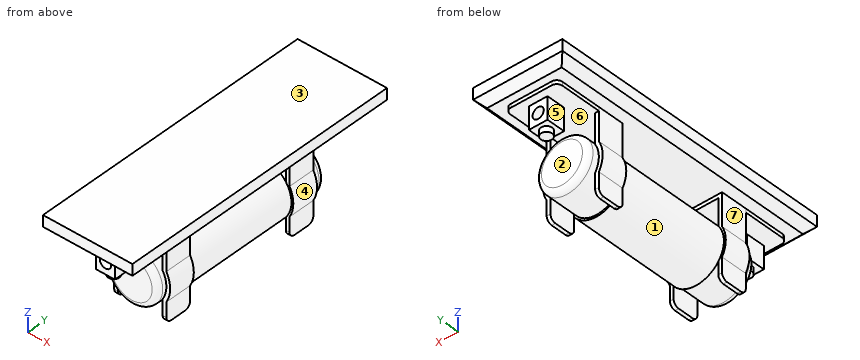
Solid Edge part; units mm, degrees
sketch "Sketch1" plane through (0, 0, 0) normal (0, -1, 0) x (1, 0, 0)
  circle A0 centre (-33.5391, 14.6196) radius 7.5
extrude "Protrusion1" add sketch "Sketch1" against normal blind 30
sketch "Sketch2" plane through (-33.5391, 0, 14.6196) normal (0, -1, 0) x (1, 0, 0)
  circle A0 centre (0, 0) radius 7
extrude "ExtrudedProtrusion_2" add sketch "Sketch2" along normal blind 9.75 and the other way blind 40.4
fillet "Round_1" radius 1.5 2 edges at (-40.5391, -9.75, 14.6196) (-40.5391, 40.4, 14.6196)
sketch "Sketch3" plane through (-33.5391, 30, 14.6196) normal (0, 1, 0) x (1, 0, 0)
  line L0 (-6, -11.6345) -> (-6, -3.6056)
  arc A0 (-6, -3.6056) -> (-6, 3.6056) centre (0, 0) cw
  line L1 (-6, 3.6056) -> (-6, 9.3463)
  line L2 (-7, 9.3463) -> (-6, 9.3463)
  line L3 (-7, 3.873) -> (-7, 9.3463)
  arc A1 (-7, -3.873) -> (-7, 3.873) centre (0, 0) cw
  line L4 (-7, -12.6345) -> (-7, -3.873)
  line L5 (7, -12.6345) -> (-7, -12.6345)
  line L6 (7, -3.873) -> (7, -12.6345)
  arc A2 (7, 3.873) -> (7, -3.873) centre (0, 0) cw
  line L7 (7, 9.3463) -> (7, 3.873)
  line L8 (6, 9.3463) -> (7, 9.3463)
  line L9 (6, 3.6056) -> (6, 9.3463)
  line L10 (6, -11.6345) -> (6, -3.6056)
  line L11 (-6, -11.6345) -> (6, -11.6345)
  arc A3 (6, 3.6056) -> (6, -3.6056) centre (0, 0) cw
extrude "ExtrudedProtrusion_3" add sketch "Sketch3" along normal blind 7.1438
sketch "Sketch4" plane through (-33.5391, 37.1438, 16.2637) normal (0, 1, 0) x (1, 0, 0)
  line L0 (7, -9.9904) -> (-7, -9.9904)
  line L1 (-7, -9.9904) -> (-7, -10.9904)
  line L2 (-7, -10.9904) -> (7, -10.9904)
  line L3 (7, -10.9904) -> (7, -9.9904)
extrude "ExtrudedProtrusion_4" add sketch "Sketch4" along normal blind 12.5
fillet "Round_2" radius 1.5 6 edges at (-40.0391, 37.1438, 5.2733) (-40.0391, 30, 5.2733) (-27.0391, 30, 5.2733) (-27.0391, 37.1438, 5.2733) (-26.5391, 49.6437, 26.7541) (-40.5391, 49.6437, 26.7541)
mirror "Mirror1" about plane through (0, 15, 0) normal (0, -1, 0) of "ExtrudedProtrusion_4", "ExtrudedProtrusion_3"
fillet "Round1" radius 1.5 6 edges at (-40.0391, -7.1438, 5.2733) (-40.0391, 0, 5.2733) (-27.0391, 0, 5.2733) (-27.0391, -7.1438, 5.2733) (-26.5391, -19.6438, 26.7541) (-40.5391, -19.6438, 26.7541)
sketch "Sketch5" plane through (-33.5391, 49.8219, 27.2541) normal (0, 0, 1) x (1, 0, 0)
  line L0 (12, 3.928) -> (12, -72.823)
  line L1 (12, -72.823) -> (-12, -72.823)
  line L2 (-12, 3.928) -> (-12, -72.823)
  line L3 (-12, 3.928) -> (12, 3.928)
  dimension "D1" = 12
extrude "ExtrudedProtrusion_7" add sketch "Sketch5" along normal blind 5
chamfer "Chamfer_1" distance 2 angle 45 4 edges at (-33.5391, 53.7499, 27.2541) (-45.5391, 15.3744, 27.2541) (-33.5391, -23.0011, 27.2541) (-21.5391, 15.3744, 27.2541)
sketch "Sketch6" plane through (-33.5391, 39.8219, 26.2541) normal (0, 0, -1) x (0, -1, 0)
  line L0 (-7.7578, -2.5) -> (-2.7578, -2.5)
  line L1 (-2.7578, -2.5) -> (-2.7578, 2.5)
  line L2 (-2.7578, 2.5) -> (-7.7578, 2.5)
  line L3 (-7.7578, 2.5) -> (-7.7578, -2.5)
  line L4 (52.4656, -2.5) -> (57.4656, -2.5)
  line L5 (57.4656, -2.5) -> (57.4656, 2.5)
  line L6 (57.4656, 2.5) -> (52.4656, 2.5)
  line L7 (52.4656, 2.5) -> (52.4656, -2.5)
extrude "ExtrudedProtrusion_8" add sketch "Sketch6" along normal blind 6
sketch "Sketch7" plane through (-33.5391, 47.5797, 22.7541) normal (0, 1, 0) x (1, 0, 0)
  circle A0 centre (0, -0.5) radius 1.5
extrude "Cutout1" cut sketch "Sketch7" against normal up to next
sketch "Sketch8" plane through (-33.5391, -17.6438, 22.7541) normal (0, -1, 0) x (-1, 0, 0)
  circle A0 centre (0, -0.5) radius 1.5
extrude "Cutout2" cut sketch "Sketch8" against normal up to next
sketch "Sketch9" plane through (-33.5391, 45.0797, 20.2541) normal (0, 0, -1) x (0, 1, 0)
  circle A0 centre (0, 0) radius 1.5
  circle A1 centre (-60.2235, 0) radius 1.5
extrude "ExtrudedProtrusion_9" add sketch "Sketch9" along normal blind 1.5
Part model, mm, in its own coordinate system. Face numbers are marked on the shaded views. A direction names the side the tool comes from. Round coordinates to 2 decimals unless told otherwise and drop trailing zeros. Write each loop counter-clockwise with the first axis right and the second up, starting at its lowest first coordinate (ties: lowest second). Pieces come first, ordered by that corner, then holes. Notation, with made-up numbers: (39.5, 60) -> (65.5, 60) arc R6 cw to (65.5, 66) -> close; hole circle Ø6 at (-30.75, 53.5). An arc over 180 degrees is marked (long way). Return JSON: item names as keys, results as strings. Group by question number.
Q1. Pin check, flat tips, straight feed: pin 1 (4.5 mm diameter, centred on y = 33.5, z = 9, fed in from +X); pin 2 (0.5 mm diameter, centred on y = 43.5, z = 26.5, fed in from -X); pin 3 (1.9 mm diameter, centred on x = -36, z = 19.5, fed in from -Y). Stop position of each tip, or through.
Q2. Saw through at A-A on y = 22. Write the cut outline in (x, z), plus the area to 3 significant figures.
Q3. Which spindle directions (+Z, -Z, +X, -X, +Y, -Y) get a long thin tool onto all of the face, cutting with end or side? Do the marked faces 4, 5, 6 and 7. Say none if no direction does.
Q4. Mould opens along Z. For the marked faces 1, 2 and 3 say: pulls with the +Z half, pulls with the -Z half, needs draft (parallel to the pull), parting line crosses it, or undercut.
Q5. Saw through at B-B on z = 28.5. Write the cut outline in (x, y) (3 decimals).
Q6. Probe L1, parallel to Y at x = -34, z = 26; L2, parallel to X at y = -5.5, z = 25.75; L3, parallel to X at y = 38.5, z = 26.75. List the from-to ranges inside material, lowest first. Write a range as [from, to].
Answer:
{
 "1": {"pin 1": "x = -26.28", "pin 2": "x = -40.54", "pin 3": "y = -17.64"},
 "2": {"outline": "(-45.54, 29.25) -> (-43.54, 27.25) -> (-23.54, 27.25) -> (-21.54, 29.25) -> (-21.54, 32.25) -> (-45.54, 32.25) -> close; circle Ø15 at (-33.54, 14.62)", "area": "293 mm2"},
 "3": {"face 4": "+X, +Y, -Y", "face 5": "-Z, -X, +Y", "face 6": "none", "face 7": "-X, +Y, -Y"},
 "4": {"face 1": "undercut", "face 2": "needs draft", "face 3": "pulls with the +Z half"},
 "5": {"outline": "(-44.785, -22.247) -> (-22.293, -22.247) -> (-22.293, 52.996) -> (-44.785, 52.996) -> close"},
 "6": {"L1": "[-17.64, -12.64], [42.58, 47.58]", "L2": "[-40.54, -39.54], [-27.54, -26.54]", "L3": "[-40.54, -26.54]"}
}
